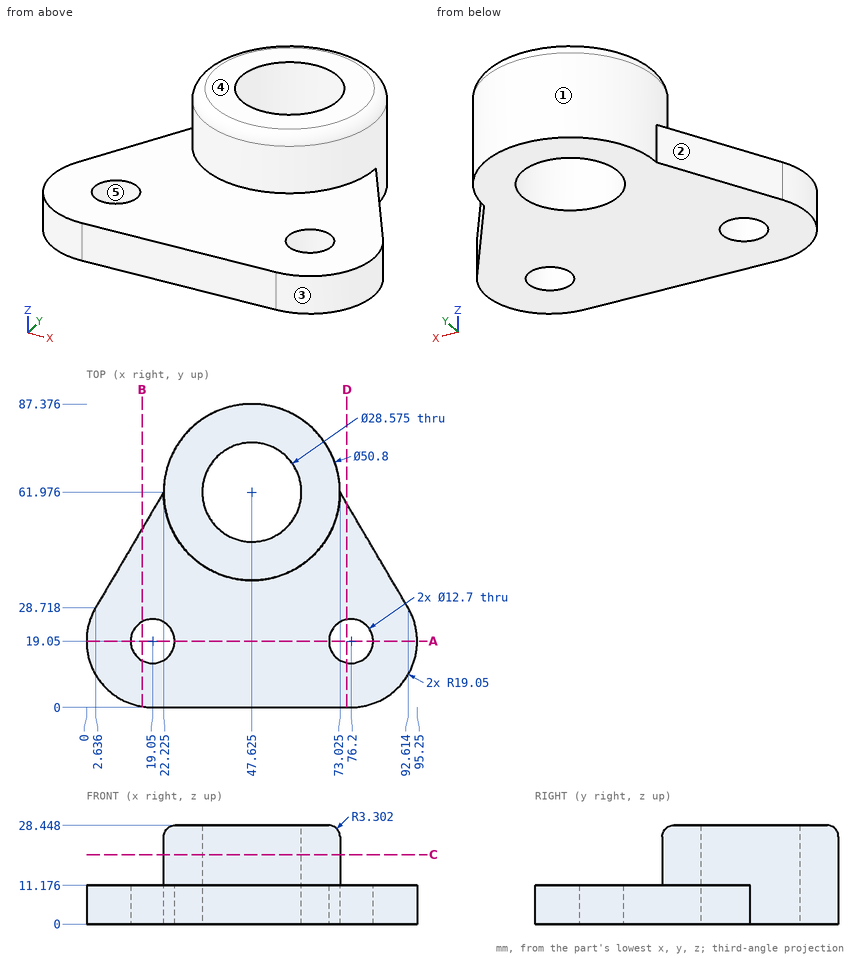
Verification items for this drawing (mm, ordinates from the low corner). A direction names the side the tool comes from. Round coordinates to 2 decimals unless told otherwise and drop trailing zeros. Order: outer loops, then holes, each group sorted by start corner. A loop starts at its lowest first (then second) coordinate and runs counter-clockwise, first axis right, second up. Notation, with made-up numbers: (-2, 47) - (32, 47) arc R25 cw to (32, 61) - close; hole circle Ø8 at (2.25, -8). An arc over 180 degrees is marked (long way). Use CSV: the item, a comma, the result in double quotes.
(1) Section check B-B on x = 16. Record the boundary of the cut face in (y, z).
Entries:
outline,"(0.25, 0) - (13.48, 0) - (13.48, 11.18) - (0.25, 11.18) - close; (24.62, 0) - (51.41, 0) - (51.41, 11.18) - (24.62, 11.18) - close"
(2) Thickness scan on probe 1 along Z at (x, y) = (83, 38); probe 2 along X at (y, z) = (61, 4); probe 3 along X at (y, z) = (66, 4.25) (1 decimal). Record the ranges inside material, lowest first. Write a range as from..to.
Entries:
probe 1,"0..11.18"
probe 2,"21.65..33.37, 61.88..73.6"
probe 3,"22.5..33.9, 61.3..72.7"
(3) Section check C-C on z = 20. Record the boundary of the cut face in (x, y) (1 decimal).
Entries:
outline,"circle Ø50.8 at (47.6, 62); hole circle Ø28.6 at (47.6, 62)"
(4) Section check D-D on x = 75. Record the boundary of the cut face in (y, z).
Entries:
outline,"(0, 0) - (12.81, 0) - (12.81, 11.18) - (0, 11.18) - close; (25.29, 0) - (58.62, 0) - (58.62, 11.18) - (25.29, 11.18) - close"
(5) Section check A-A on y = 19.05. Record the boundary of the cut face in (x, z).
Entries:
outline,"(0, 0) - (12.7, 0) - (12.7, 11.18) - (0, 11.18) - close; (25.4, 0) - (69.85, 0) - (69.85, 11.18) - (25.4, 11.18) - close; (82.55, 0) - (95.25, 0) - (95.25, 11.18) - (82.55, 11.18) - close"
(6) Access from +Z, -Z, +X, -X, +Y, -Y to the whole of each face (thin tool, end or side, straight path). Record for the marked faces 1 and 2.
Entries:
face 1,"+Z"
face 2,"+Z, -Z, -X, +Y"
(7) Gauge pin test, flat ends, axial feed: pin 1 Ø1.5 at (x, z) = (44, 15.5) entering from +Y; pin 2 Ø1.5 at (y, z) = (71, 18) entering from -X; pin 3 Ø11.5 at (x, y) = (19.05, 19.05) entering from -Z; pin 4 Ø6 at (y, z) = (9, 10) entering from -X. Record the tip position at first contact, or that the pin passes through.
Entries:
pin 1,"y = 87.21"
pin 2,"x = 23.61"
pin 3,"through"
pin 4,"x = 1.35"
(8) Mould release check, pull along X, two halves, no side actions. Record for the marked faces 3, 4 and 5: released by +X, released by -X, zero draft, split by the parting line, or undercut.
Entries:
face 3,"released by +X"
face 4,"zero draft"
face 5,"undercut"
